from build123d import *

# Parameters (mm, degrees)
SKICA1_W                = 60
SKICA1_H                = 4.6
P_IDAT_VYSUNUT_M1_DEPTH = 0.9
SKICA2_R                = 1.85
P_IDAT_VYSUNUT_M2_DEPTH = 2
ZAOBLIT1_R              = 0.4


with BuildPart() as part:
    # Skica1 → Přidat vysunutím1 (new body)
    with BuildSketch(Plane.XY):
        Rectangle(SKICA1_W, SKICA1_H)
    extrude(amount=P_IDAT_VYSUNUT_M1_DEPTH)

    # Skica2 → Přidat vysunutím2 (add)
    with BuildSketch(Plane.XY.offset(0.9)):
        with Locations((-5, 0)):
            Circle(SKICA2_R)
    extrude(amount=P_IDAT_VYSUNUT_M2_DEPTH)

    # Zaoblit1
    zaoblit1_edges = [part.edges().sort_by_distance(p)[0] for p in [
        (-6.85, 0, 2.9),
    ]]
    fillet(zaoblit1_edges, radius=ZAOBLIT1_R)


solid = part.part
Build history of the part. All positions in model axes, mm. A direction names the side the tool comes from. Coordinates: 2 decimals unless noted, no trailing zeros. Order: outer loops, then holes, each group sorted by start corner. A loop starts at its lowest first (then second) coordinate and runs counter-clockwise, first axis right, second up. Notation, with made-up numbers: (39.5, 46) - (75.5, 46) arc R27 ccw to (75.5, 75) - close; hole circle Ø1 at (-4, 85.5). An arc over 180 degrees is marked (long way). Write each question's results on one line, items separated by ' | '. Start each with the question number.
Item 1: Flat gauge pin, fed straight in: pin 1 (1 mm diameter, centred on y = 1.5, z = 2, fed in from +X). Where does the tip first touch, or does it go through?
Item 2: Band-saw the part on A-A on y = 0. Write the cut outline in (x, z), and give its area (3 significant figures).
Item 3: Wall check: probe 1 along X at (y, z) = (0.1, 2.15); probe 2 along Z at (x, y) = (4, -1.9); probe 3 along X at (y, z) = (-0.9, 1.1). Give the ranges that are in metal, low to high. Write a range as [from, to].
Item 4: Band-saw the part on C-C on z = 1.9. Write the cut outline in (x, y).
Item 5: Tool access for faces 1 (the face through (-6.85, 0.08, 1.69)), 2 (the face through (-5, 0, 2.9)): list every direction of +Z, -Z, +X, -X, +Y, -Y with a clear straight run to the whole face (end or side of a thin tool).
Item 6: Band-saw the part on B-B on x = -5. Write the cut outline in (y, z), and give its area (3 significant figures).
Numbers:
1) pin 1: x = -3.44
2) outline: (-30, 0) - (30, 0) - (30, 0.9) - (-3.15, 0.9) - (-3.15, 2.5) arc R0.4 ccw to (-3.55, 2.9) - (-6.45, 2.9) arc R0.4 ccw to (-6.85, 2.5) - (-6.85, 0.9) - (-30, 0.9) - close | area: 61.3 mm^2
3) probe 1: [-6.85, -3.15] | probe 2: [0, 0.9] | probe 3: [-6.62, -3.38]
4) outline: circle Ø3.7 at (-5, 0)
5) face 1: +Z | face 2: +Z, +X, -X, +Y, -Y
6) outline: (-2.3, 0) - (2.3, 0) - (2.3, 0.9) - (1.85, 0.9) - (1.85, 2.5) arc R0.4 ccw to (1.45, 2.9) - (-1.45, 2.9) arc R0.4 ccw to (-1.85, 2.5) - (-1.85, 0.9) - (-2.3, 0.9) - close | area: 11.5 mm^2
